from build123d import *

# Parameters (mm, degrees)
F1_DEPTH = 25
F2_R     = 2.95
F3_DEPTH = 10
F4_R     = 3
F5_R     = 2
F8_R     = 10.709349
F8_R_2   = 9.209349
F9_DEPTH = 2


with BuildPart() as f1:
    # F0 (on Front) → F1 (new body)
    with BuildSketch(Plane.XZ):
        Polygon((13.40901, 18), (0, 0), (-13.40901, 18), (-15.40901, 18), (-15.40901, -7), (15.40901, -7), (15.40901, 18), align=None)
    extrude(amount=F1_DEPTH)

    # F2 (on face) → F3 (join)
    with BuildSketch(Plane(origin=(0, 0, -7), x_dir=(1, 0, 0), z_dir=(0, 0, -1))):
        with Locations((0, 12.5)):
            Circle(F2_R)
    extrude(amount=F3_DEPTH)

    # F4
    f4_edges = [f1.edges().sort_by_distance(p)[0] for p in [
        (-13.40901, -12.5, 18),
        (13.40901, -12.5, 18),
    ]]
    fillet(f4_edges, radius=F4_R)

    # F5
    f5_edges = [f1.edges().sort_by_distance(p)[0] for p in [
        (0, -12.5, 0),
    ]]
    fillet(f5_edges, radius=F5_R)

    # F8 (on face) → F9 (cut, symmetric)
    with BuildSketch(Plane(origin=(0, -12.5, 0), x_dir=(-1, 0, 0), z_dir=(0, 1, 0))):
        with Locations((0, 5.47572)):
            Circle(F8_R)
        with Locations((0, 5.47572)):
            Circle(F8_R_2, mode=Mode.SUBTRACT)
    extrude(amount=F9_DEPTH, both=True, mode=Mode.SUBTRACT)


solid = f1.part
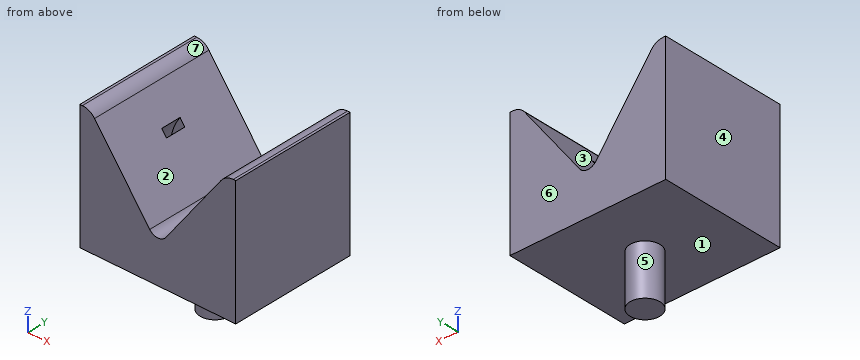
Design review of the part built by this model. Coordinates are the model's own, in mm. Face numbers are marked on the shaded views. A direction names the side the tool comes from. Coordinates: 2 decimals unless noted, no trailing zeros. Write each loop counter-clockwise with the first axis right and the second up, starting at its lowest first coordinate (ties: lowest second). Pieces come first, ordered by that corner, then holes. Notation, with made-up numbers: (31.5, 25.5) - (76.5, 25.5) arc R24 ccw to (76.5, 40.5) - close; hole circle Ø5 at (23, -37). An arc over 180 degrees is marked (long way). One line per item, written item: value.
1) Insertion check: pin 1 (4 mm diameter, centred on x = 1.5, y = -7, fed in from -Z); pin 2 (13.5 mm diameter, centred on x = 4.5, z = 0.5, fed in from +Y); pin 3 (1.5 mm diameter, centred on x = -2, y = -19.5, fed in from +Z). Each pin has a flat end and moves straight along its axis. Give the tip position at first contact, or say it passes through.
Answer sheet:
pin 1: stops at z = -7
pin 2: stops at y = 0
pin 3: stops at z = 3.69
2) Add section A-A (x = 0). State the section outline as (y, z) points, plus the area to 3 significant figures.
Answer sheet:
outline: (-25, -7) - (-15.45, -7) - (-15.45, -17) - (-9.55, -17) - (-9.55, -7) - (0, -7) - (0, 1.35) - (-25, 1.35) - close; hole (-14.5, -5.23) - (-10.5, -5.23) - (-10.5, -3.73) - (-14.5, -3.73) - close
area: 262 mm2
3) Add section B-B (z = 8). State the section outline as (x, y) points, plus the area to 3 significant figures.
Answer sheet:
outline: (-15.41, -25) - (-5.96, -25) - (-5.96, 0) - (-15.41, 0) - close; (5.96, -25) - (15.41, -25) - (15.41, 0) - (5.96, 0) - close; hole (-10.41, -14.5) - (-8.86, -14.5) - (-8.86, -10.5) - (-10.41, -10.5) - close; hole (8.86, -14.5) - (10.41, -14.5) - (10.41, -10.5) - (8.86, -10.5) - close
area: 460 mm2
4) Add section D-D (z = 14.5). State the section outline as (x, y) points, plus the area to 3 significant figures.
Answer sheet:
outline: (-15.41, -25) - (-10.8, -25) - (-10.8, 0) - (-15.41, 0) - close; (10.8, -25) - (15.41, -25) - (15.41, 0) - (10.8, 0) - close
area: 230 mm2
5) For the marked faces 5, 6 and 7, list the 3-axis set-ups (+Z, -Z, +X, -X, +Y, -Y) from which the entire face can be reached by the end or side of a thin tool; tool diameter is ignored.
Answer sheet:
face 5: -Z
face 6: +Z, -Z, +X, -X, +Y
face 7: +Z, +Y, -Y
6) Mouldability with a two-part tool opening along X and no side actions: class the marked faces 1, 2, 3 and 4 as +X half, -X half, draft (parallel to the pull), parting line (faces both ways), or undercut.
Answer sheet:
face 1: draft
face 2: undercut
face 3: undercut
face 4: -X half
7) To check wall thickness, follow probe 1 along Z at (x, y) = (0, -11.85); probe 2 along X at (y, z) = (-11.5, 6); probe 3 along X at (y, z) = (-12.5, 8). State the ranges of each line that lie inside material, in increasing order.
Answer sheet:
probe 1: z = -17 to -5.23, -3.73 to 1.35
probe 2: x = -15.41 to -10.7, -9.19 to -4.47, 4.47 to 9.19, 10.7 to 15.41
probe 3: x = -15.41 to -10.41, -8.86 to -5.96, 5.96 to 8.86, 10.41 to 15.41
8) Add section C-C (y = -3). State the section outline as (x, z) points.
Answer sheet:
outline: (-15.41, -7) - (15.41, -7) - (15.41, 18) - (14.92, 18) arc R3 ccw to (12.51, 16.79) - (1.6, 2.15) arc R2 cw to (-1.6, 2.15) - (-12.51, 16.79) arc R3 ccw to (-14.92, 18) - (-15.41, 18) - close
